Model file for the job. Use its own axes, mm. A direction names the side the tool comes from. Round coordinates to 2 decimals unless told otherwise and drop trailing zeros. Order: outer loops, then holes, each group sorted by start corner. A loop starts at its lowest first (then second) coordinate and runs counter-clockwise, first axis right, second up. Notation, with made-up numbers: (-14.75, 76) - (22.25, 76) arc R23 ccw to (22.25, 91) - close; hole circle Ø1 at (-31, -23). An arc over 180 degrees is marked (long way). Put each result on its own line as item: value. Start each with the question number.
Item 1: Probe probe 1 along X at (y, z) = (3.6, -119); probe 2 along X at (y, z) = (0.5, -104); probe 3 along Z at (x, y) = (-59, 1.3). List the from-to ranges inside material, lowest first.
Item 2: Which spindle directions (+Z, -Z, +X, -X, +Y, -Y) get a long thin tool onto all of the face, cutting with end or side? Do faces 1 (the face through (-66.35, 4.33, 201.5)), 2 (the face through (-65.594, 2.226, 200.719)), 3 (the face through (68.32, 4.36, 203.14)). Say none if no direction does.
Item 3: Saw through at B-B on y = 2.6. List the corners of the cut face in (x, z), plus the area to 3 significant figures.
Item 4: Mould opens along X. For faces 4 (the face through (-68.14, 0.14, -203.32)), 5 (the face through (-67.4, 3.67, -202.57)), 6 (the face through (-69, 0, 1)) say: pulls with the +X half, pulls with the -X half, needs draft (parallel to the pull), parting line crosses it, or undercut.
Autodesk Inventor part; units mm, degrees
ref_plane "YZ Plane" through (0, 0, 0) normal (1, 0, 0) x (0, 1, 0)
ref_plane "XZ Plane" through (0, 0, 0) normal (0, 1, 0) x (-1, 0, 0)
ref_plane "XY Plane" through (0, 0, 0) normal (0, 0, 1) x (1, 0, 0)
sketch "Sketch1" plane through (0, 0, 0) normal (0, 1, 0) x (-1, 0, 0)
  circle A0 centre (60, 195) radius 12
  circle A1 centre (60, -195) radius 12
  circle A2 centre (-60, 195) radius 12
  circle A3 centre (-60, -195) radius 12
  line L0 (72, 195) -> (72, -195)
  line L1 (60, -207) -> (-60, -207)
  line L2 (60, 207) -> (-60, 207)
  line L3 (-72, 195) -> (-72, -195)
  line L4 (68, 195) -> (68, -195)
  circle A4 centre (60, 195) radius 8
  line L5 (60, 203) -> (-60, 203)
  circle A5 centre (-60, 195) radius 8
  line L6 (-68, 195) -> (-68, -195)
  circle A6 centre (-60, -195) radius 8
  line L7 (60, -203) -> (-60, -203)
  circle A7 centre (60, -195) radius 8
  point P0 (0, 0)
  point P1 (72, 0)
  point P2 (0, 207)
  point P3 (35, 143)
  point P4 (68, 135)
  point P5 (68, -135)
  point P6 (35, -143)
  point P7 (-60, -203)
  point P8 (-68, -135)
  point P9 (-68, 135)
  point P10 (-60, 203)
  dimension "d0" = 24
  dimension "d1" = 24
  dimension "d2" = 24
  dimension "d3" = 24
  dimension "d6" = 4
  dimension "d7" = 4
  dimension "d8" = 4
  dimension "d9" = 4
  dimension "d10" = 4
  dimension "d11" = 4
  dimension "d12" = 4
  dimension "d13" = 4
  dimension "d35" = 414
  dimension "d36" = 144
extrude "Extrusion1" add sketch "Sketch1" along normal blind 4.5 contours A0 L4 A4 L5 | L0 A1 L4 A0 | A0 L5 A2 L2 | A1 L7 A7 L4 | A2 L5 A5 L6 | L1 A3 L7 A1 | A2 L6 A3 L3 | A3 L6 A6 L7 picked at (54.6594, 203.5636) picked at (54.6594, -203.5636) picked at (-54.6594, 203.5636) picked at (-54.6594, -203.5636)
sketch "Sketch2" plane through (0, 4.5, 0) normal (0, 1, 0) x (1, 0, 0)
  line L0 (-72, 195) -> (-72, -195)
  arc A0 (-72, -195) -> (-60, -207) centre (-60, -195) ccw
  line L1 (-60, -207) -> (60, -207)
  arc A1 (60, -207) -> (72, -195) centre (60, -195) ccw
  line L2 (72, -195) -> (72, 195)
  arc A2 (72, 195) -> (60, 207) centre (60, 195) ccw
  line L3 (60, 207) -> (-60, 207)
  arc A3 (-60, 207) -> (-72, 195) centre (-60, 195) ccw
  line L4 (-69.5, -195) -> (-69.5, 195)
  arc A4 (-60, 204.5) -> (-69.5, 195) centre (-60, 195) ccw
  line L5 (-60, 204.5) -> (60, 204.5)
  arc A5 (69.5, 195) -> (60, 204.5) centre (60, 195) ccw
  line L6 (69.5, 195) -> (69.5, -195)
  arc A6 (60, -204.5) -> (69.5, -195) centre (60, -195) ccw
  line L7 (60, -204.5) -> (-60, -204.5)
  arc A7 (-69.5, -195) -> (-60, -204.5) centre (-60, -195) ccw
  line L8 (-70.5, -195) -> (-70.5, 195)
  arc A8 (-60, 205.5) -> (-70.5, 195) centre (-60, 195) ccw
  line L9 (-60, 205.5) -> (60, 205.5)
  arc A9 (70.5, 195) -> (60, 205.5) centre (60, 195) ccw
  line L10 (70.5, 195) -> (70.5, -195)
  arc A10 (60, -205.5) -> (70.5, -195) centre (60, -195) ccw
  line L11 (60, -205.5) -> (-60, -205.5)
  arc A11 (-70.5, -195) -> (-60, -205.5) centre (-60, -195) ccw
  point P0 (0, 0)
  dimension "d16" = 2.5
  dimension "d17" = 1.5
extrude "Extrusion2" cut sketch "Sketch2" against normal blind 1 contours L8 A8 L9 A9 L10 A10 L11 A11
chamfer "Chamfer3" distance 0.5 distance2 1 8 edges at (0, 4.5, 205.5) (-67.4246, 4.5, 202.4246) (-70.5, 4.5, 0) (-67.4246, 4.5, -202.4246) (0, 4.5, -205.5) (67.4246, 4.5, -202.4246) (70.5, 4.5, 0) (67.4246, 4.5, 202.4246) measured on face at (-71, 4.5, 65)
chamfer "Chamfer4" distance 0.5 distance2 1 8 edges at (0, 4.5, 204.5) (66.7175, 4.5, 201.7175) (69.5, 4.5, 0) (66.7175, 4.5, -201.7175) (0, 4.5, -204.5) (-66.7175, 4.5, -201.7175) (-69.5, 4.5, 0) (-66.7175, 4.5, 201.7175) measured on face at (-69, 4.5, -65)
chamfer "Chamfer5" distance 0.5 angle 45 32 edges at (0, 4.5, 207) (68.4853, 4.5, 203.4853) (72, 4.5, 0) (68.4853, 4.5, -203.4853) (0, 4.5, -207) (-68.4853, 4.5, -203.4853) (-72, 4.5, 0) (-68.4853, 4.5, 203.4853) (0, 4.5, 203) (-65.6569, 4.5, 200.6569) (-68, 4.5, 0) (-65.6569, 4.5, -200.6569) (0, 4.5, -203) (65.6569, 4.5, -200.6569) (68, 4.5, 0) (65.6569, 4.5, 200.6569) (68.4853, 0, 203.4853) (72, 0, 0) (68.4853, 0, -203.4853) (0, 0, -207) (-68.4853, 0, -203.4853) (-72, 0, 0) (-68.4853, 0, 203.4853) (0, 0, 207) (0, 0, 203) (-65.6569, 0, 200.6569) (-68, 0, 0) (-65.6569, 0, -200.6569) (0, 0, -203) (65.6569, 0, -200.6569) (68, 0, 0) (65.6569, 0, 200.6569)
properties part number "LI0005-SEAL"
Results found:
1. probe 1: x = -72 to -70.55, -69.45 to -68, 68 to 69.45, 70.55 to 72
1. probe 2: x = -72 to -68, 68 to 72
1. probe 3: z = -207 to -203, 203 to 207
2. face 1: +Y
2. face 2: +Y, -Y
2. face 3: +Z, +X, +Y
3. outline: (-72, -195) arc R12 ccw to (-60, -207) - (60, -207) arc R12 ccw to (72, -195) - (72, 195) arc R12 ccw to (60, 207) - (-60, 207) arc R12 ccw to (-72, 195) - close; hole (-68, -195) arc R8 ccw to (-60, -203) - (60, -203) arc R8 ccw to (68, -195) - (68, 195) arc R8 ccw to (60, 203) - (-60, 203) arc R8 ccw to (-68, 195) - close
3. area: 4,330 mm²
4. face 4: pulls with the -X half
4. face 5: undercut
4. face 6: needs draft
